Can you work these out from the model? Positions are in its coordinate system, mm. A direction names the side the tool comes from. Round coordinates to 2 decimals unless told otherwise and drop trailing zeros. Loops run counter-clockwise (first coordinate to the right, second up) from the corner with the lowest first, then second, coordinate; pieces in that order, holes last. Notation, with made-up numbers: (11, 77) - (26, 77) arc R20 cw to (26, 93) - close; hole circle Ø11 at (67.25, 22.25). An arc over 180 degrees is marked (long way). Answer as CSV lines item,"result".
```python
from build123d import *

# Parameters (mm, degrees)
SZKIC2_R                    = 4
SZKIC2_R_2                  = 32.5
DODANIE_WYCI_GNI_CIE1_DEPTH = 10
WYTNIJ_WYCI_GNI_CIE1_DEPTH  = 4
WYTNIJ_WYCI_GNI_CIE2_START  = -10
WYTNIJ_WYCI_GNI_CIE2_DEPTH  = 1741.763240958
DODANIE_WYCI_GNI_CIE2_START = -10
SZKIC4_R                    = 32.5
SZKIC4_R_2                  = 30.5
DODANIE_WYCI_GNI_CIE2_DEPTH = 3
ZAOKR_GLENIE1_R             = 60
ZAOKR_GLENIE2_R             = 8
ZAOKR_GLENIE3_R             = 3


with BuildPart() as part:
    # Szkic2 → Dodanie-wyci_gni_cie1 (new body)
    with BuildSketch(Plane(origin=(0, 0, 0), x_dir=(1, 0, 0), z_dir=(0, 1, 0))):
        with BuildLine():
            Line((1543.993451292, -292.693431604), (1602.649516269, -405.490665796))
            ThreePointArc((1602.649516269, -405.490665796), (1610.447293462, -409.078792342), (1615.858300195, -402.415385751))
            Line((1615.858300195, -402.415385751), (1618.512976907, -281.976412469))
            Line((1618.512976907, -281.976412469), (1680.947289281, -153.356819868))
            ThreePointArc((1680.947289281, -153.356819868), (1678.976293723, -144.796984225), (1670.19309755, -144.902220776))
            Line((1670.19309755, -144.902220776), (1554.640194786, -240.313313752))
            ThreePointArc((1554.640194786, -240.313313752), (1540.051589656, -264.620128285), (1543.993451292, -292.693431604))
        make_face()
        with Locations(Location((1608.86, -402.261131492, 0), (0, 0, 270))):
            Circle(SZKIC2_R, mode=Mode.SUBTRACT)
        with Locations(Location((1581.69995966, -273.085544755, 0), (0, 0, 270))):
            Circle(SZKIC2_R_2, mode=Mode.SUBTRACT)
        with Locations(Location((1674.65, -150.3, 0), (0, 0, 270))):
            Circle(SZKIC2_R, mode=Mode.SUBTRACT)
    extrude(amount=DODANIE_WYCI_GNI_CIE1_DEPTH)

    # Szkic3 → Wytnij-wyci_gni_cie1 (cut)
    with BuildSketch(Plane(origin=(0, 10, 0), x_dir=(1, 0, 0), z_dir=(0, 1, 0))):
        with BuildLine():
            Line((1666.310350061, -161.316546708), (1605.842827281, -241.193195468))
            ThreePointArc((1605.842827281, -241.193195468), (1615.649420401, -251.932906257), (1620.968093066, -265.468872331))
            Line((1620.968093066, -265.468872331), (1668.654089364, -167.231970482))
            ThreePointArc((1668.654089364, -167.231970482), (1668.783849398, -163.758542263), (1666.310350061, -161.316546708))
        make_face()
        with BuildLine():
            Line((1662.025493572, -162.020782011), (1575.342850703, -233.593935954))
            ThreePointArc((1575.342850703, -233.593935954), (1591.370558871, -234.272151308), (1605.842827281, -241.193195468))
            Line((1605.842827281, -241.193195468), (1666.310350061, -161.316546708))
            ThreePointArc((1666.310350061, -161.316546708), (1664.072870869, -161.090335403), (1662.025493572, -162.020782011))
        make_face()
        with BuildLine():
            Line((1562.06257658, -307.933402448), (1602.825740378, -386.322093118))
            ThreePointArc((1602.825740378, -386.322093118), (1607.801974735, -388.611894192), (1611.255066167, -384.359570486))
            Line((1611.255066167, -384.359570486), (1613.16331738, -297.784879179))
            ThreePointArc((1613.16331738, -297.784879179), (1589.491721347, -312.31931146), (1562.06257658, -307.933402448))
        make_face()
    extrude(amount=-WYTNIJ_WYCI_GNI_CIE1_DEPTH, mode=Mode.SUBTRACT)

    # Szkic3_3 → Wytnij-wyci_gni_cie2 (cut, through all)
    with BuildSketch(Plane(origin=(0, 10, 0), x_dir=(1, 0, 0), z_dir=(0, 1, 0)).offset(WYTNIJ_WYCI_GNI_CIE2_START)):
        with BuildLine():
            Line((1662.025493572, -162.020782011), (1575.342850703, -233.593935954))
            ThreePointArc((1575.342850703, -233.593935954), (1591.370558871, -234.272151308), (1605.842827281, -241.193195468))
            Line((1605.842827281, -241.193195468), (1666.310350061, -161.316546708))
            ThreePointArc((1666.310350061, -161.316546708), (1664.072870869, -161.090335403), (1662.025493572, -162.020782011))
        make_face()
        with BuildLine():
            Line((1666.310350061, -161.316546708), (1605.842827281, -241.193195468))
            ThreePointArc((1605.842827281, -241.193195468), (1615.649420401, -251.932906257), (1620.968093066, -265.468872331))
            Line((1620.968093066, -265.468872331), (1668.654089364, -167.231970482))
            ThreePointArc((1668.654089364, -167.231970482), (1668.783849398, -163.758542263), (1666.310350061, -161.316546708))
        make_face()
        with BuildLine():
            Line((1562.06257658, -307.933402448), (1602.825740378, -386.322093118))
            ThreePointArc((1602.825740378, -386.322093118), (1607.801974735, -388.611894192), (1611.255066167, -384.359570486))
            Line((1611.255066167, -384.359570486), (1613.16331738, -297.784879179))
            ThreePointArc((1613.16331738, -297.784879179), (1589.491721347, -312.31931146), (1562.06257658, -307.933402448))
        make_face()
    extrude(amount=WYTNIJ_WYCI_GNI_CIE2_DEPTH, mode=Mode.SUBTRACT)

    # Szkic4 → Dodanie-wyci_gni_cie2 (add)
    with BuildSketch(Plane(origin=(0, 0, 0), x_dir=(-1, 0, 0), z_dir=(0, -1, 0)).offset(DODANIE_WYCI_GNI_CIE2_START)):
        with Locations(Location((-1581.69995966, -273.085544755, 0), (0, 0, 90))):
            Circle(SZKIC4_R)
        with Locations(Location((-1581.69995966, -273.085544755, 0), (0, 0, 90))):
            Circle(SZKIC4_R_2, mode=Mode.SUBTRACT)
    extrude(amount=DODANIE_WYCI_GNI_CIE2_DEPTH)

    # Zaokr_glenie1
    zaokr_glenie1_edges = [part.edges().sort_by_distance(p)[0] for p in [
        (1618.512976907, 5, 281.976412469),
    ]]
    fillet(zaokr_glenie1_edges, radius=ZAOKR_GLENIE1_R)

    # Zaokr_glenie2
    zaokr_glenie2_edges = [part.edges().sort_by_distance(p)[0] for p in [
        (1575.342850703, 3, 233.593935954),
        (1562.06257658, 5, 307.933402448),
    ]]
    fillet(zaokr_glenie2_edges, radius=ZAOKR_GLENIE2_R)

    # Zaokr_glenie3
    zaokr_glenie3_edges = [part.edges().sort_by_distance(p)[0] for p in [
        (1620.968093066, 3, 265.468872331),
        (1613.16331738, 5, 297.784879179),
    ]]
    fillet(zaokr_glenie3_edges, radius=ZAOKR_GLENIE3_R)


solid = part.part
```
Q1. Imagine slicing it at C-C (x = 1596). Write out the boundary of the cut face in (y, z), then the cut area to 3 significant figures.
Checks:
outline,"(0, 206.16) - (10, 206.16) - (10, 216.54) - (0, 216.54) - close; (0, 235.73) - (10, 235.73) - (10, 246.15) - (7, 246.15) - (7, 243.9) - (0, 243.9) - close; (0, 302.27) - (7, 302.27) - (7, 300.03) - (10, 300.03) - (10, 310.44) - (0, 310.44) - close; (0, 373.2) - (10, 373.2) - (10, 392.7) - (0, 392.7) - close"
area,"476 mm²"
Q2. If I drill on line 1 along Z through (x, y) = (1608, 2.25); line 2 along X through (y, z) = (5.5, 258); line 3 along Z through (x, y) = (1594.5, 8.75), over which ranges is the centre line in solid material (lowest first)? Write a range as [from, to].
Checks:
line 1,"[196.25, 206.63], [242.95, 253.99], [292.18, 303.22], [388.56, 398.35], [406.17, 409.21]"
line 2,"[1541.97, 1552.91], [1610.49, 1618.75], [1624.59, 1630.15]"
line 3,"[207.4, 217.78], [235.19, 245.4], [300.77, 310.98], [370.31, 389.82]"
Q3. Imagine slicing it at A-A (z = 201). Write out the boundary of the cut face in (x, y).
Checks:
outline,"(1602.25, 0) - (1614.82, 0) - (1614.82, 10) - (1602.25, 10) - close; (1652.26, 0) - (1657.82, 0) - (1657.82, 10) - (1652.26, 10) - close"
Q4. On a 3-axis mill with a long thin cutter (end or side, diameter ignored), from which of +Z, -Z, +X, -X, +Y, -Y can I reach the whole of each face in a straight line? I mean faces 1 (the flat face through (1616, 10, 277)), 2 (the flat face through (1586.56, 4.93, 355.04)). Say none if no direction works.
Checks:
face 1,"+Z, -Z, +X, -X, +Y"
face 2,"+Y, -Y"
Q5. Imagine slicing it at B-B (x = 1674.65). Write out the boundary of the cut face in (y, z).
Checks:
outline,"(0, 143.3) - (10, 143.3) - (10, 146.3) - (0, 146.3) - close; (0, 154.3) - (10, 154.3) - (10, 166.33) - (0, 166.33) - close"
Q6. Imagine slicing it at D-D (y = 5). Write out the boundary of the cut face in (x, z), then the cut area to 3 significant figures.
Checks:
outline,"(1543.99, 292.69) arc R42.5 ccw to (1554.64, 240.31) - (1670.19, 144.9) arc R7 ccw to (1680.95, 153.36) - (1624.23, 270.19) arc R60 cw to (1618.22, 295.07) - (1615.86, 402.42) arc R7 ccw to (1602.65, 405.49) - close; hole circle Ø65 at (1581.7, 273.09); hole (1570.74, 324.62) arc R8 ccw to (1578.48, 312.96) arc R40 cw to (1608.02, 303.21) arc R3 ccw to (1612.99, 305.53) - (1611.26, 384.36) arc R4.47 ccw to (1602.83, 386.32) - close; hole (1590.6, 221) - (1662.03, 162.02) arc R4.31 ccw to (1668.65, 167.23) - (1624.35, 258.5) arc R3 ccw to (1618.87, 258.3) arc R40 cw to (1593.36, 234.82) arc R8 ccw to start; hole circle Ø8 at (1608.86, 402.26); hole circle Ø8 at (1674.65, 150.3)"
area,"5,510 mm²"
Q7. We'd pull the mould along X, two halves only. Please class faces 3 (the cylindrical face through (1619.93, 5.07, 282.13)), 4 (the cylindrical face through (1540.134, 4.93, 264.224)), 5 (the cylindrical face through (1549.973, 3.451, 266.04)): pulls with the +X half, pulls with the -X half, needs draft (parallel to the pull), parting line crosses it, or undercut.
Checks:
face 3,"pulls with the +X half"
face 4,"pulls with the -X half"
face 5,"undercut"
Q8. I'm going to push flat-ended pins straight in: pin 1 Ø5 at (x, z) = (1674.65, 150.3) entering from +Y; pin 2 Ø3 at (y, z) = (5, 246.5) entering from +X; pin 3 Ø2 at (x, y) = (1634.5, 9) entering from -Z; pin 4 Ø1.5 at (y, z) = (1.5, 335) entering from -X. Where does each tip first touch, or does it pass through?
Checks:
pin 1,"through"
pin 2,"x = 1636.46"
pin 3,"z = 173.55"
pin 4,"x = 1565.6"
